```python
from build123d import *

# Parameters (mm, degrees)
ESQUISSE1_R             = 10.85
ESQUISSE1_R_2           = 9
BOSS_EXTRU_1_DEPTH      = 7
ESQUISSE2_R             = 18
BOSS_EXTRU_2_DEPTH      = 2
ESQUISSE4_R             = 18
BOSS_EXTRU_3_DEPTH      = 8
BOSS_EXTRU_3_TAPER      = 51.5
ESQUISSE5_R             = 1.5
ENL_V_MAT_EXTRU_1_DEPTH = 4
ESQUISSE6_R             = 3.9
ENL_V_MAT_EXTRU_2_DEPTH = 8
ESQUISSE9_R             = 10.85
ENL_V_MAT_EXTRU_4_DEPTH = 7
ESQUISSE10_R            = 9
ENL_V_MAT_EXTRU_5_DEPTH = 8


with BuildPart() as part:
    # Esquisse1 → Boss.-Extru.1 (new body)
    with BuildSketch(Plane(origin=(0, 0, 0), x_dir=(1, 0, 0), z_dir=(0, 1, 0))):
        with Locations(Location((0, 0, 0), (0, 0, 270))):
            Circle(ESQUISSE1_R)
        with Locations(Location((0, 0, 0), (0, 0, 270))):
            Circle(ESQUISSE1_R_2, mode=Mode.SUBTRACT)
    extrude(amount=BOSS_EXTRU_1_DEPTH)

    # Esquisse2 → Boss.-Extru.2 (add)
    with BuildSketch(Plane(origin=(0, 7, 0), x_dir=(1, 0, 0), z_dir=(0, 1, 0))):
        with Locations(Location((0, 0, 0), (0, 0, 270))):
            Circle(ESQUISSE2_R)
    extrude(amount=BOSS_EXTRU_2_DEPTH)

    # Esquisse4 → Boss.-Extru.3 (add)
    with BuildSketch(Plane(origin=(0, 9, 0), x_dir=(1, 0, 0), z_dir=(0, 1, 0))):
        with Locations(Location((0, 0, 0), (0, 0, 270))):
            Circle(ESQUISSE4_R)
    extrude(amount=BOSS_EXTRU_3_DEPTH, taper=BOSS_EXTRU_3_TAPER)

    # Esquisse5 → Enlèv. mat.-Extru.1 (cut)
    with BuildSketch(Plane.XZ.offset(-7)):
        with Locations(Location((-12.898733794, 8.041309999, 0), (0, 0, 270))):
            Circle(ESQUISSE5_R)
        with Locations(Location((13.413345636, 7.149976143, 0), (0, 0, 270))):
            Circle(ESQUISSE5_R)
        with Locations(Location((-0.514611842, -15.191286142, 0), (0, 0, 270))):
            Circle(ESQUISSE5_R)
    extrude(amount=-ENL_V_MAT_EXTRU_1_DEPTH, mode=Mode.SUBTRACT)

    # Esquisse6 → Enlèv. mat.-Extru.2 (cut)
    with BuildSketch(Plane(origin=(0, 17, 0), x_dir=(1, 0, 0), z_dir=(0, 1, 0))):
        with Locations((-0.514611842, 15.191286142)):
            Circle(ESQUISSE6_R)
        with Locations((13.413345636, -7.149976143)):
            Circle(ESQUISSE6_R)
        with Locations((-12.898733794, -8.041309999)):
            Circle(ESQUISSE6_R)
    extrude(amount=-ENL_V_MAT_EXTRU_2_DEPTH, mode=Mode.SUBTRACT)

    # Esquisse9 → Enlèv. mat.-Extru.4 (cut)
    with BuildSketch(Plane.XZ):
        Circle(ESQUISSE9_R)
    extrude(amount=-ENL_V_MAT_EXTRU_4_DEPTH, mode=Mode.SUBTRACT)

    # Esquisse10 → Enlèv. mat.-Extru.5 (cut)
    with BuildSketch(Plane.XZ.offset(-7)):
        with Locations(Location((0, 0, 0), (0, 0, 270))):
            Circle(ESQUISSE10_R)
    extrude(amount=-ENL_V_MAT_EXTRU_5_DEPTH, mode=Mode.SUBTRACT)


solid = part.part
```
Can you work these out from the model? Positions are in its coordinate system, mm. A direction names the side the tool comes from. Coordinates: 2 decimals unless noted, no trailing zeros. Loops run counter-clockwise (first coordinate to the right, second up) from the corner with the lowest first, then second, coordinate; pieces in that order, holes last. Notation, with made-up numbers: M 19,54 L 24,54 A27 ccw 24,81 Z; hole C 48.25,72 d8. An arc over 180 degrees is marked long. Put each result on its own line as item: value. Start each with the question number.
(1) Imagine slicing it at B-B on y = 13.5. List the corners of the cut face in (x, z) for me, and give its area (3 significant figures).
(2) Imagine slicing it at D-D on y = 15.75. List the corners of the cut face in (x, z) for me.
(3) Which directions (+Z, -Z, +X, -X, +Y, -Y) give clear straight access to the entire face, cutting with the end or side of a thin tool? Please do faces 1 (the face through (12.839, 7.986, 5.764)), 2 (the face through (-11, 9, 8)), 3 (the face through (0, 15, 0)).
(4) We'd pull the mould along Z, two halves only. Please class faces 4 (the face through (2.532, 16.612, 8.042)), 5 (the face through (0, 17, 0)), 6 (the face through (2.703, 10.944, -8.584)): +Z half, -Z half, draft (parallel to the pull), parting line (faces both ways), or undercut.
(5) Imagine slicing it at A-A on z = 0. List the corners of the cut face in (x, y) for me.
(6) Imagine slicing it at C-C on y = 11. List the corners of the cut face in (x, z) for me.
(7) I need wall thicknesses on probe 1 along X at (y, z) = (7.5, 8); probe 2 along X at (y, z) = (14.75, 6.5); probe 3 along Y at (x, z) = (-2, 0.5). Which ranges of each line are inside material? Lowest first, please.
(8) Will these pins go through, and if not, where does the flat tip stop? pin 1 Ø7.5 at (x, z) = (1.5, -14) entering from +Y; pin 2 Ø5 at (y, z) = (11, 3) entering from -X; pin 3 Ø1.8 at (x, z) = (-0.51, -15.19) entering from -Y; pin 4 Ø3.5 at (x, z) = (-12.9, 8.04) entering from +Y.
Worked answers:
1. outline: M -11.54,4.39 A12.34 ccw -2.79,-12.02 A3.9 cw 1.97,-12.18 A12.34 ccw 11.81,3.6 A3.9 cw 9.57,7.8 A12.34 ccw -9.02,8.43 A3.9 cw Z; hole C 0,0 d18
1. area: 214 mm2
2. outline: C 0,0 d19.03
3. face 1: +Y, -Y
3. face 2: +Y
3. face 3: -Y
4. face 4: parting line
4. face 5: draft
4. face 6: undercut
5. outline: M -18,7 L -9,7 L -9,15 L 9,15 L 9,7 L 18,7 L 18,9 L 7.94,17 L -7.94,17 L -18,9 Z
6. outline: M -14.78,4.62 A15.49 ccw -4.4,-14.85 A3.9 cw 3.38,-15.11 A15.49 ccw 15.06,3.61 A3.9 cw 11.39,10.49 A15.49 ccw -10.66,11.23 A3.9 cw Z; hole C 0,0 d18
7. probe 1: x = -16.12 to -14.4, -11.4 to -4.12, 4.12 to 12.18, 14.65 to 16.12
7. probe 2: x = -8.59 to -6.22, 6.22 to 8.59
7. probe 3: y = 15 to 17
8. pin 1: stops at y = 15.1
8. pin 2: stops at x = -17.94
8. pin 3: passes through
8. pin 4: stops at y = 9
